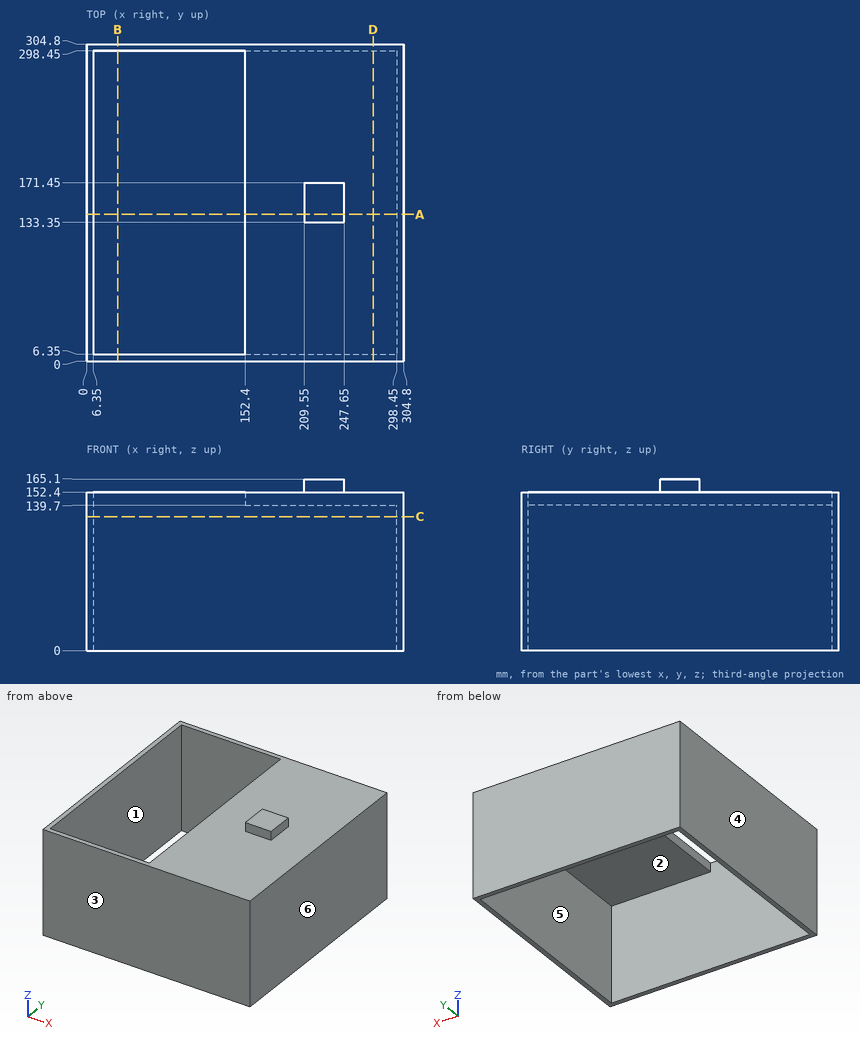
Could you check a few things on this drawing? It's one solid part, dimensions in mm from its lowest x, y, z. A direction names the side the tool comes from. Round coordinates to 2 decimals unless told otherwise and drop trailing zeros. Loops run counter-clockwise (first coordinate to the right, second up) from the corner with the lowest first, then second, coordinate; pieces in that order, holes last. Notation, with made-up numbers: M 22.25,30.25 L 36.25,30.25 A12 ccw 36.25,38.25 Z; hole C -17.75,-14.5 d6. An arc over 180 degrees is marked long. Write each question's results on one line, items separated by ' | '. Start each with the question number.
(1) I want a section at C-C (z = 129). Please give me the cut outline in (x, y), then the cut area to 3 significant figures.
(2) I want a section at A-A (y = 141). Please give me the cut outline in (x, z).
(3) Thinking about a two-plate mould opening in Y: for the marked faces 1, 2, 3 and 4, which applies, pulls with the +Y half, pulls with the -Y half, needs draft (parallel to the pull), parting line crosses it, or undercut?
(4) I want a section at D-D (x = 275.5). Please give me the cut outline in (y, z).
(5) If I drill on probe 1 along Y at (x, z) = (27.5, 132.5); probe 2 along X at (y, z) = (269.5, 147.5), over which ranges is the centre line in solid material (lowest first)? Write a range as from..to.
(6) Will these pins go through, and if not, where does the flat tip stop? P1, Ø6.5, axis at x = 237.5, z = 158.5, coming from the +Y side; P2, Ø10, axis at y = 159, z = 160, coming from the -X side; P3, Ø3, axis at x = 177, y = 58, coming from the -Z side.
(7) On a 3-axis mill with a long thin cutter (end or side, diameter ignored), from which of +Z, -Z, +X, -X, +Y, -Y can I reach the whole of each face in a straight line? I mean the marked faces 5 and 6. Say none if no direction works.
(8) I want a section at B-B (x = 30). Please give me the cut outline in (y, z).
Solved:
1) outline: M 0,0 L 304.8,0 L 304.8,304.8 L 0,304.8 Z; hole M 6.35,6.35 L 298.45,6.35 L 298.45,298.45 L 6.35,298.45 Z | area: 7,580 mm²
2) outline: M 0,0 L 6.35,0 L 6.35,152.4 L 0,152.4 Z; M 152.4,139.7 L 298.45,139.7 L 298.45,0 L 304.8,0 L 304.8,152.4 L 247.65,152.4 L 247.65,165.1 L 209.55,165.1 L 209.55,152.4 L 152.4,152.4 Z
3) face 1: undercut | face 2: undercut | face 3: pulls with the -Y half | face 4: needs draft
4) outline: M 0,0 L 6.35,0 L 6.35,139.7 L 298.45,139.7 L 298.45,0 L 304.8,0 L 304.8,152.4 L 0,152.4 Z
5) probe 1: y = 0..6.35, 298.45..304.8 | probe 2: x = 0..6.35, 152.4..304.8
6) P1: stops at y = 171.45 | P2: stops at x = 209.55 | P3: stops at z = 139.7
7) face 5: -Z | face 6: +Z, -Z, +X, +Y, -Y
8) outline: M 0,0 L 6.35,0 L 6.35,152.4 L 0,152.4 Z; M 298.45,0 L 304.8,0 L 304.8,152.4 L 298.45,152.4 Z
